Could you check a few things on this model? Use its own coordinates, in mm. A direction names the side the tool comes from. Coordinates: 2 decimals unless noted, no trailing zeros. Write each loop counter-clockwise with the first axis right and the second up, starting at its lowest first coordinate (ties: lowest second). Pieces come first, ordered by that corner, then holes. Notation, with made-up numbers: M -25.75,46.5 L 21.25,46.5 A19 cw 21.25,72.5 Z; hole C -37.75,-29.5 d1. An arc over 180 degrees is marked long. Write item = value, one per line.
Autodesk Inventor part; units mm, degrees
ref_plane "YZ Plane" through (0, 0, 0) normal (1, 0, 0) x (0, 1, 0)
ref_plane "XZ Plane" through (0, 0, 0) normal (0, 1, 0) x (-1, 0, 0)
ref_plane "XY Plane" through (0, 0, 0) normal (0, 0, 1) x (1, 0, 0)
sketch "Sketch1" plane through (0, 0, 0) normal (0, 1, 0) x (-1, 0, 0)
  line L0 (-26.9875, 42.8625) -> (26.9875, 42.8625)
  line L1 (26.9875, 42.8625) -> (26.9875, -42.8625)
  line L2 (26.9875, -42.8625) -> (-26.9875, -42.8625)
  line L3 (-26.9875, -42.8625) -> (-26.9875, 42.8625)
  line L4 (-26.9875, 42.8625) -> (26.9875, -42.8625) construction
  line L5 (26.9875, 42.8625) -> (-26.9875, -42.8625) construction
  point P0 (0, 0)
  dimension "d0" = 53.975
  dimension "d1" = 85.725
extrude "Extrusion1" add sketch "Sketch1" along normal blind 1.57
sketch "Sketch2" plane through (0, 1.57, 0) normal (0, 1, 0) x (1, 0, 0)
  line L0 (-26.9875, -42.8625) -> (26.9875, -42.8625)
  line L1 (-26.9875, 42.8625) -> (-26.9875, -42.8625)
  line L2 (26.9875, 42.8625) -> (-26.9875, 42.8625)
  line L3 (26.9875, -42.8625) -> (26.9875, 42.8625)
  point P0 (0, 0)
  point P1 (-22.9235, -38.7985)
  point P2 (-22.9235, 38.7985)
  point P3 (22.9235, 38.7985)
  dimension "d4" = 4.064
  dimension "d5" = 4.064
  dimension "d6" = 4.064
  dimension "d7" = 4.064
  dimension "d8" = 4.064
  dimension "d9" = 4.064
hole "Hole1" at (-22.9235, 1.57, 38.7985) at (-22.9235, 1.57, -38.7985) at (22.9235, 1.57, -38.7985) direction (0, -1, 0) diameter 3 depth 2.54
sketch "Sketch3" plane through (0, 1.57, 0) normal (0, 1, 0) x (1, 0, 0)
  line L0 (26.9875, -42.8625) -> (26.9875, 42.8625)
  line L1 (26.9875, 42.8625) -> (-26.9875, 42.8625)
  line L2 (16.9065, 28.2465) -> (10.9065, 28.2465)
  line L3 (10.9065, 28.2465) -> (10.9065, 42.7465)
  line L4 (10.9065, 42.7465) -> (16.9065, 42.7465)
  line L5 (16.9065, 42.7465) -> (16.9065, 28.2465)
  line L6 (16.9065, 28.2465) -> (10.9065, 42.7465) construction
  line L7 (10.9065, 28.2465) -> (16.9065, 42.7465) construction
  point P0 (0, 0)
  point P1 (13.9065, 35.4965)
  dimension "d17" = 13.081
  dimension "d18" = 7.366
  dimension "d19" = 14.5
  dimension "d20" = 6
extrude "Extrusion2" add sketch "Sketch3" along normal blind 5
sketch "Sketch4" plane through (16.9065, 1.57, -42.7465) normal (0, 0, -1) x (-1, 0, 0)
  line L0 (6, 0) -> (6, 5)
  circle A0 centre (3, 2.5) radius 2.5
  point P0 (16.9065, -1.57)
  dimension "d23" = 5
extrude "Extrusion3" add sketch "Sketch4" along normal blind 2.5
sketch "Sketch5" plane through (0, 1.57, 0) normal (0, 1, 0) x (1, 0, 0)
  line L0 (-26.9875, -42.8625) -> (26.9875, -42.8625)
  line L1 (26.9875, -42.8625) -> (26.9875, 42.8625)
  line L2 (-4.9284, -30.8693) -> (-9.1184, -30.8693)
  line L3 (-9.1184, -30.8693) -> (-9.1184, -36.0693)
  line L4 (-9.1184, -36.0693) -> (-4.9284, -36.0693)
  line L5 (-4.9284, -36.0693) -> (-4.9284, -30.8693)
  line L6 (-4.9284, -30.8693) -> (-9.1184, -36.0693) construction
  line L7 (-9.1184, -30.8693) -> (-4.9284, -36.0693) construction
  point P0 (0, 0)
  point P1 (-7.3025, -33.9725)
  point P2 (-7.0234, -33.4693)
  dimension "d26" = 8.89
  dimension "d27" = 34.29
  dimension "d28" = 5.2
  dimension "d29" = 4.19
extrude "Extrusion4" add sketch "Sketch5" along normal blind 8.77
sketch "Sketch6" plane through (0, 1.57, 0) normal (0, 1, 0) x (1, 0, 0)
  line L0 (-6.0004, 7.1846) -> (-24.0004, 7.1846)
  line L1 (-24.0004, 7.1846) -> (-24.0004, 32.6846)
  line L2 (-24.0004, 32.6846) -> (-6.0004, 32.6846)
  line L3 (-6.0004, 32.6846) -> (-6.0004, 7.1846)
  line L4 (-6.0004, 7.1846) -> (-24.0004, 32.6846) construction
  line L5 (-24.0004, 7.1846) -> (-6.0004, 32.6846) construction
  point P0 (0, 0)
  point P1 (-15.0004, 19.9346)
  dimension "d34" = 25.5
  dimension "d35" = 18
extrude "Extrusion5" add sketch "Sketch6" along normal blind 4.2
sketch "Sketch7" plane through (0, 0, 0) normal (0, -1, 0) x (1, 0, 0)
  line L0 (2.7595, 37.1835) -> (-3.1405, 37.1835)
  line L1 (-3.1405, 37.1835) -> (-3.1405, 41.6835)
  line L2 (-3.1405, 41.6835) -> (2.7595, 41.6835)
  line L3 (2.7595, 41.6835) -> (2.7595, 37.1835)
  line L4 (2.7595, 37.1835) -> (-3.1405, 41.6835) construction
  line L5 (-3.1405, 37.1835) -> (2.7595, 41.6835) construction
  line L6 (-26.9875, 42.8625) -> (26.9875, 42.8625)
  line L7 (-26.9875, -42.8625) -> (-26.9875, 42.8625)
  line L8 (26.9875, 42.8625) -> (26.9875, -42.8625)
  point P0 (0, 0)
  point P1 (-0.1905, 39.4335)
  dimension "d36" = 4.5
  dimension "d37" = 5.9
  dimension "d38" = 3.429
  dimension "d40" = 27.178
extrude "Extrusion6" add sketch "Sketch7" along normal blind 6
sketch "Sketch8" plane through (0, 1.57, 0) normal (0, 1, 0) x (1, 0, 0)
  line L0 (26.0985, -42.6085) -> (16.2941, -42.6085)
  line L1 (16.2941, -42.6085) -> (16.2941, -32.7279)
  line L2 (16.2941, -32.7279) -> (26.0985, -32.7279)
  line L3 (26.0985, -32.7279) -> (26.0985, -42.6085)
  line L4 (26.0985, -42.6085) -> (16.2941, -32.7279) construction
  line L5 (16.2941, -42.6085) -> (26.0985, -32.7279) construction
  line L6 (26.9875, -42.8625) -> (26.9875, 42.8625)
  line L7 (-26.9875, -42.8625) -> (26.9875, -42.8625)
  point P0 (0, 0)
  point P1 (21.1963, -37.6682)
  dimension "d43" = 9.8044
  dimension "d44" = 9.8806
  dimension "d45" = 0.889
  dimension "d46" = 0.254
extrude "Extrusion7" add sketch "Sketch8" along normal blind 6.1722
sketch "Sketch9" plane through (16.2941, 1.57, 42.6085) normal (0, 0, 1) x (1, 0, 0)
  line L0 (0, 0) -> (0, 6.1722)
  line L1 (7.0358, 4.2799) -> (2.2606, 4.2799)
  line L2 (2.2606, 4.2799) -> (2.2606, 1.8923)
  line L3 (2.2606, 1.8923) -> (7.0358, 1.8923)
  line L4 (7.0358, 1.8923) -> (7.0358, 4.2799)
  line L5 (7.0358, 4.2799) -> (2.2606, 1.8923) construction
  line L6 (2.2606, 4.2799) -> (7.0358, 1.8923) construction
  line L7 (0, 6.1722) -> (9.8044, 6.1722)
  point P0 (-16.2941, -1.57)
  point P1 (4.6482, 3.0861)
  dimension "d52" = 3.0861
  dimension "d53" = 2.2606
extrude "Extrusion8" add sketch "Sketch9" along normal blind 2.4892
sketch "Sketch10" plane through (0, 1.57, 0) normal (0, 1, 0) x (1, 0, 0)
  line L0 (26.9875, -42.8625) -> (26.9875, 42.8625)
  line L1 (-26.9875, -42.8625) -> (26.9875, -42.8625)
  line L2 (13.0175, -42.2275) -> (5.3975, -42.2275)
  line L3 (5.3975, -42.2275) -> (5.3975, -37.1475)
  line L4 (5.3975, -37.1475) -> (13.0175, -37.1475)
  line L5 (13.0175, -37.1475) -> (13.0175, -42.2275)
  line L6 (13.0175, -42.2275) -> (5.3975, -37.1475) construction
  line L7 (5.3975, -42.2275) -> (13.0175, -37.1475) construction
  point P0 (0, 0)
  point P1 (9.2075, -39.6875)
  dimension "d56" = 17.78
  dimension "d57" = 3.175
  dimension "d58" = 7.62
  dimension "d59" = 5.08
extrude "Extrusion9" add sketch "Sketch10" along normal blind 1.8
properties part number "ECG PCB"
Item 1: Imagine slicing it at C-C (x = -1). Write out the boundary of the cut face in (y, z).
Numbers:
outline = M -6,37.18 L 0,37.18 L 0,-42.86 L 1.57,-42.86 L 1.57,42.86 L 0,42.86 L 0,41.68 L -6,41.68 Z
Item 2: I'm going to push flat-ended pins straight in: P1, Ø4.5, axis at x = -14.5, y = 4, coming from the -Z side; P2, Ø5, axis at x = 19, y = 3, coming from the -Z side; P3, Ø4, axis at y = 8.5, z = -35.5, coming from the -X side. Where does each tip first touch, or does it pass through?
Numbers:
P1 = -32.68
P2 = -42.86
P3 = 10.91
Item 3: If we mould it in two halves opening along Y, with no side actions, what happens to faces 1 (the face through (16.906, 4, -36)), 2 (the face through (21, 3, 42.608)), 3 (the face through (21, 7.742, 38))? For each: pulls with the +Y half, pulls with the -Y half, needs draft (parallel to the pull), parting line crosses it, or undercut.
Numbers:
face_1 = needs draft
face_2 = undercut
face_3 = pulls with the +Y half
Item 4: If I drill on line 1 along X through (y, z) = (2.25, -30.5); line 2 along Z through (x, y) = (12, 1); line 3 along X through (y, z) = (3.25, 41.5), over which ranges is the centre line in solid material (lowest first)?
Numbers:
line_1 = -24 to -6, 10.91 to 16.91
line_2 = -42.86 to 42.86
line_3 = 5.4 to 13.02, 16.29 to 26.1
Item 5: For faces 4 (the face through (-6, 4, -20)), 5 (the face through (16.294, 5, 38)), 6 (the face through (-7, 6, 36.069)), 7 (the face through (2.76, -3, 39)), 8 (the face through (-4.928, 6, 34)), which set-ups out of +Z, -Z, +X, -X, +Y, -Y let a thin tool reach every point of the face, with its end or its side?
Numbers:
face_4 = -Z, +Y
face_5 = +Z, +Y
face_6 = +Z, -X, +Y
face_7 = +Z, -Z, +X, -Y
face_8 = +Z, -Z, +Y
Item 6: Imagine slicing it at D-D (z = 4.5). Write out the boundary of the cut face in (x, y), and give its area (3 significant figures).
Numbers:
outline = M -26.99,0 L 26.99,0 L 26.99,1.57 L -26.99,1.57 Z
area = 84.7 mm²
Item 7: Imagine slicing it at A-A (x = -20). Write out the boundary of the cut face in (y, z), and give its area (3 significant figures).
Numbers:
outline = M 0,-42.86 L 1.57,-42.86 L 1.57,-32.68 L 5.77,-32.68 L 5.77,-7.18 L 1.57,-7.18 L 1.57,42.86 L 0,42.86 Z
area = 242 mm²
Item 8: Imagine slicing it at B-B (y = -4.5). Write out the boundary of the cut face in (x, z).
Numbers:
outline = M -3.14,37.18 L 2.76,37.18 L 2.76,41.68 L -3.14,41.68 Z
